```python
from build123d import *

# Parameters (mm, degrees)
F0_R          = 11
F0_R_2        = 10
F1_DEPTH      = 1000
F3_DEPTH      = 15
F3_DEPTH_BACK = 15


with BuildPart() as f1:
    # F0 (on Front) → F1 (new body)
    with BuildSketch(Plane.XZ):
        Circle(F0_R)
        Circle(F0_R_2, mode=Mode.SUBTRACT)
    extrude(amount=F1_DEPTH)

    # F2 (on Top) → F3 (join, two sides)
    with BuildSketch(Plane.XY) as f3_sk:
        Polygon((-15, -515), (15, -515), (15, -485), (0, -485), (-15, -485), align=None)
    extrude(amount=F3_DEPTH)
    extrude(f3_sk.sketch, amount=-F3_DEPTH_BACK)


solid = f1.part
```
Geometry: final body of the model. Coordinates: model frame, mm. A direction names the side the tool comes from. Round coordinates to 2 decimals unless told otherwise and drop trailing zeros. Write each loop counter-clockwise with the first axis right and the second up, starting at its lowest first coordinate (ties: lowest second). Pieces come first, ordered by that corner, then holes. Notation, with made-up numbers: (-33.75, -8) -> (-19.75, -8) arc R16 cw to (-19.75, -3) -> close; hole circle Ø9 at (89, 56.25). An arc over 180 degrees is marked (long way). Return JSON: item names as keys, results as strings.
Q1. First-contact query: pin 1 Ø16 at (x, z) = (3, 0) entering from +Y; pin 2 Ø4 at (y, z) = (-102.5, -7.5) entering from -X; pin 3 Ø10 at (x, z) = (3, -1.5) entering from -Y; pin 4 Ø1.5 at (y, z) = (-445.5, 7) entering from +X. Flat tips, straight axial feed; report the tip coordinate or a pass-through.
From the geometry:
{"pin 1": "y = 0", "pin 2": "x = -9.53", "pin 3": "y = -515", "pin 4": "x = 9.05"}
Q2. Set-up query: faces 5 (the flat face through (7, -485, 10)), 6 (the flat face through (0, -500, 15)), 7 (the flat face through (-7, -515, 10)). Return all of +Z, -Z, +X, -X, +Y, -Y with unobstructed straight access to the full face (end or side cutting, diameter ignored); none if empty.
From the geometry:
{"face 5": "+Y", "face 6": "+Z, +X, -X, +Y, -Y", "face 7": "-Y"}
Q3. Section C-C on y = -448. Return the cut outline in (x, z), and give its area (3 significant figures).
From the geometry:
{"outline": "circle Ø22 at (0, 0); hole circle Ø20 at (0, 0)", "area": "66.0 mm2"}
Q4. Ray query, line 1 (X direction, y = -720.5, z = 0); line 2 (X direction, y = -420, z = 1). Return the intervals inside material, ascending.
From the geometry:
{"line 1": "-11 to -10, 10 to 11", "line 2": "-10.95 to -9.95, 9.95 to 10.95"}
Q5. Mould query, pull axis Z, two halves, no side actions, for faces 1 (the cylindrical face through (-2.17, -239.1, -9.76)), 2 (the flat face through (0, -500, -15)), 3 (the cylindrical face through (-2.38, -239.1, -10.74)), 4 (the flat face through (15, -500, 0)). Classes: +Z half, -Z half, draft (parallel to the pull), parting line (faces both ways), or undercut.
From the geometry:
{"face 1": "undercut", "face 2": "-Z half", "face 3": "parting line", "face 4": "draft"}
Q6. Section B-B on x = 0. Return the cut outline in (y, z).
From the geometry:
{"outline": "(-1000, -11) -> (-515, -11) -> (-515, -15) -> (-485, -15) -> (-485, -11) -> (0, -11) -> (0, -10) -> (-485, -10) -> (-485, 10) -> (0, 10) -> (0, 11) -> (-485, 11) -> (-485, 15) -> (-515, 15) -> (-515, 11) -> (-1000, 11) -> (-1000, 10) -> (-515, 10) -> (-515, -10) -> (-1000, -10) -> close"}
Q7. Section A-A on z = 0. Return the cut outline in (x, y).
From the geometry:
{"outline": "(-15, -515) -> (-11, -515) -> (-11, -1000) -> (-10, -1000) -> (-10, -515) -> (10, -515) -> (10, -1000) -> (11, -1000) -> (11, -515) -> (15, -515) -> (15, -485) -> (11, -485) -> (11, 0) -> (10, 0) -> (10, -485) -> (-10, -485) -> (-10, 0) -> (-11, 0) -> (-11, -485) -> (-15, -485) -> close"}
